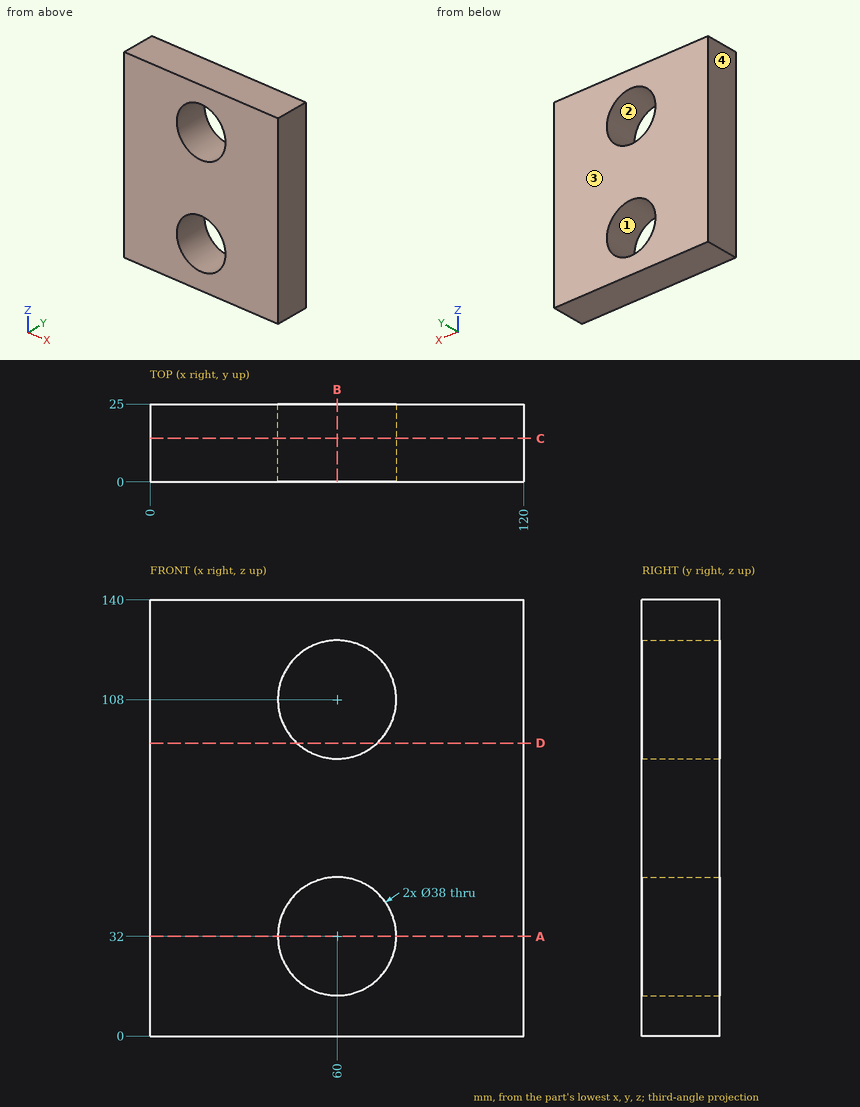
The figure shows three views and two pictorial views of one solid part (mm, origin at its lowest corner). Answer the questions. Coordinates: 2 decimals unless noted, no trailing zeros. Loops run counter-clockwise (first coordinate to the right, second up) from the corner with the lowest first, then second, coordinate; pieces in that order, holes last. Notation, with made-up numbers: (33.5, -26.75) - (39.5, -26.75) arc R20 ccw to (39.5, -17.75) - close; hole circle Ø7 at (25, 2). An arc over 180 degrees is marked (long way). Answer in a Markdown table with one row per item.
Q1. Straight lines are drawn through the part: line 1 along Z through (x, y) = (60, 16); line 2 along Z through (x, y) = (65, 20.5); line 3 along X through (y, z) = (21, 94). For each, find the intervals that lie inside material, in ascending order. Write a range as [from, to].
Here are the results:
| item | result |
|---|---|
| line 1 | z = [0, 13], [51, 89], [127, 140] |
| line 2 | z = [0, 13.67], [50.33, 89.67], [126.33, 140] |
| line 3 | x = [0, 47.15], [72.85, 120] |
Q2. Find section D-D on z = 94. Write down the section's boundary in (x, y).
Here are the results:
| item | result |
|---|---|
| outline | (0, 0) - (47.15, 0) - (47.15, 25) - (0, 25) - close; (72.85, 0) - (120, 0) - (120, 25) - (72.85, 25) - close |
Q3. Find section C-C on y = 14. Write down the section's boundary in (x, z), plus the area to 3 significant figures.
Here are the results:
| item | result |
|---|---|
| outline | (0, 0) - (120, 0) - (120, 140) - (0, 140) - close; hole circle Ø38 at (60, 32); hole circle Ø38 at (60, 108) |
| area | 14,500 mm^2 |
Q4. Given P1, Ø4, axis at x = 47, z = 39.5, coming from the +Y side, flat-ended and moving along its own axis, determine where the tip first touches the part or whether it passes through.
Here are the results:
| item | result |
|---|---|
| P1 | passes through |
Q5. The mould has two halves that part along X. Classify the marked faces 1, 2, 3 and 4: pulls with the +X half, pulls with the -X half, needs draft (parallel to the pull), parting line crosses it, or undercut.
Here are the results:
| item | result |
|---|---|
| face 1 | undercut |
| face 2 | undercut |
| face 3 | needs draft |
| face 4 | pulls with the -X half |
Q6. Find section A-A on z = 32. Write down the section's boundary in (x, y), plus the area to 3 significant figures.
Here are the results:
| item | result |
|---|---|
| outline | (0, 0) - (41, 0) - (41, 25) - (0, 25) - close; (79, 0) - (120, 0) - (120, 25) - (79, 25) - close |
| area | 2,050 mm^2 |
Q7. Find section B-B on x = 60. Write down the section's boundary in (y, z), plus the area to 3 significant figures.
Here are the results:
| item | result |
|---|---|
| outline | (0, 0) - (25, 0) - (25, 13) - (0, 13) - close; (0, 51) - (25, 51) - (25, 89) - (0, 89) - close; (0, 127) - (25, 127) - (25, 140) - (0, 140) - close |
| area | 1,600 mm^2 |
